Verification items for the finished model (mm, model axes). A direction names the side the tool comes from. Coordinates: 2 decimals unless noted, no trailing zeros. Loops run counter-clockwise (first coordinate to the right, second up) from the corner with the lowest first, then second, coordinate; pieces in that order, holes last. Notation, with made-up numbers: (16, 20.25) - (68, 20.25) arc R25 ccw to (68, 59.25) - close; hole circle Ø7 at (-32, 6). An arc over 180 degrees is marked (long way). Answer as CSV lines item,"result". Start each with the question number.
1. Cross-section at A-A (x = 0). Enter the section's corners in (y, z), plus the area to 3 significant figures.
2. Gauge pin test, flat ends, axial feed: P1, Ø0.6, axis at x = -12.5, z = -2, coming from the +Y side; P2, Ø1.2, axis at y = -1, z = -3, coming from the +X side; P3, Ø0.6, axis at x = 13, z = -3.5, coming from the +Y side. Record the tip position at first contact, or that the pin passes through.
3. Release check for a two-part mould opening along Y. For faces 1 (the flat face through (13, -2, -3)), 2 (the cylindrical face through (9.8, -10, -3.1)), 3 (the flat face through (6, -6, 0)) record: pulls with the +Y half, pulls with the -Y half, needs draft (parallel to the pull), parting line crosses it, or undercut.
4. Set-up check for faces 4 (the flat face through (2, 13, -3)), 5 (the cylindrical face through (-9.8, 10, -3.1)), 6 (the flat face through (-12, 0, -3)), 7 (the flat face through (2, -13, -3)): record each of +Z, -Z, +X, -X, +Y, -Y from which the full face is reachable in a straight line by a thin tool's end or side.
5. Cross-section at C-C (z = -3.5). Enter the section's corners in (x, y), plus the area to 3 significant figures.
6. Material ranges on line 1 (Y direction, x = 0, z = -5.5); line 2 (Y direction, x = -1, z = -2); line 3 (Z direction, x = -10.75, y = -7.75), recorded low to high. Write a range as [from, to].
```python
from build123d import *

# Parameters (mm, degrees)
SKETCH1_R        = 14
SKETCH1_R_2      = 6.188
BASENUT_DEPTH    = 8
CHAMFER1_SIZE    = 0.5
ENDCHAMFER_SIZE  = 0.866025404
ENDCHAMFER_SIZE2 = 0.5
CHAMFER2_SIZE    = 0.7
SLOTCUT_DEPTH    = 27.474268868
SLOTPAT_COUNT    = 4


with BuildPart() as part:
    # Sketch1 → BaseNut (new body)
    with BuildSketch(Plane.XY):
        Circle(SKETCH1_R)
        Circle(SKETCH1_R_2, mode=Mode.SUBTRACT)
    extrude(amount=-BASENUT_DEPTH)

    # Sketch2 → StepCut (revolve, cut)
    with BuildSketch(Plane(origin=(0, 0, 0), x_dir=(1, 0, 0), z_dir=(0, 1, 0)), mode=Mode.PRIVATE) as stepcut_sk:
        Polygon((-14, 8), (-10, 8), (-14, 5.690598923), align=None)
    revolve(stepcut_sk.sketch.rotate(Axis((0, 0, -4.560481664), (0, 0, 1)), 180), axis=Axis((0, 0, -4.560481664), (0, 0, 1)), mode=Mode.SUBTRACT)

    # Chamfer1
    chamfer1_edges = [part.edges().sort_by_distance(p)[0] for p in [
        (-14, 0, 0),
    ]]
    chamfer(chamfer1_edges, length=CHAMFER1_SIZE)

    # EndChamfer
    endchamfer_edges = [part.edges().sort_by_distance(p)[0] for p in [
        (-6.188, 0, 0),
    ]]
    endchamfer_side = [part.faces().sort_by_distance(p)[0] for p in [
        (-13.118162338, 0, 0),
    ]]
    chamfer(endchamfer_edges, length=ENDCHAMFER_SIZE, length2=ENDCHAMFER_SIZE2, reference=endchamfer_side[0])

    # Chamfer2
    chamfer2_edges = [part.edges().sort_by_distance(p)[0] for p in [
        (-6.188, 0, -8),
    ]]
    chamfer(chamfer2_edges, length=CHAMFER2_SIZE)

    # Sketch3 → SlotCut (cut, through all)
    with BuildSketch(Plane(origin=(-3.554280188, 4.131027526, -8), x_dir=(-1, 0, 0), z_dir=(0, 0, -1))):
        with BuildLine():
            Line((-5.554280188, -16.131027526), (-1.554280188, -16.131027526))
            Line((-1.554280188, -16.131027526), (-1.554280188, -17.987433987))
            ThreePointArc((-1.554280188, -17.987433987), (-3.554280188, -18.131027526), (-5.554280188, -17.987433987))
            Line((-5.554280188, -17.987433987), (-5.554280188, -16.131027526))
        make_face()
    slotcut = extrude(amount=-SLOTCUT_DEPTH, mode=Mode.SUBTRACT)

    # SlotPat: SlotCut ×4 about axis
    slotpat_axis = Axis((0, 0, -4.560481664), (0, 0, 1))
    for i in range(1, SLOTPAT_COUNT):
        add(slotcut.rotate(slotpat_axis, i * 360 / SLOTPAT_COUNT), mode=Mode.SUBTRACT)


solid = part.part
```
Values follow:
1,outline,"(-12, -6.85) - (-10, -8) - (-6.89, -8) - (-6.19, -7.3) - (-6.19, -0.5) - (-7.05, 0) - (-12, 0) - close; (6.19, -7.3) - (6.89, -8) - (10, -8) - (12, -6.85) - (12, 0) - (7.05, 0) - (6.19, -0.5) - close"
1,area,"89.8 mm²"
2,P1,"stops at y = 6.87"
2,P2,"stops at x = 12"
2,P3,"stops at y = 5.89"
3,face 1,"undercut"
3,face 2,"pulls with the -Y half"
3,face 3,"needs draft"
4,face 4,"+Z, -Z, +Y"
4,face 5,"+Z, -Z, -X, +Y"
4,face 6,"+Z, -Z, -X"
4,face 7,"+Z, -Z, -Y"
5,outline,"(-13.86, -2) arc R14 ccw to (-2, -13.86) - (-2, -12) - (2, -12) - (2, -13.86) arc R14 ccw to (13.86, -2) - (12, -2) - (12, 2) - (13.86, 2) arc R14 ccw to (2, 13.86) - (2, 12) - (-2, 12) - (-2, 13.86) arc R14 ccw to (-13.86, 2) - (-12, 2) - (-12, -2) - close; hole circle Ø12.38 at (0, 0)"
5,area,"464 mm²"
6,line 1,"y = [-12, -6.19], [6.19, 12]"
6,line 2,"y = [-12, -6.11], [6.11, 12]"
6,line 3,"z = [-6.12, 0]"
